Answer from the drawing. Dimensions are ordinates in mm from the lowest x, y and z of the part. Round coordinates to 2 decimals unless told otherwise and drop trailing zeros. Loops run counter-clockwise (first coordinate to the right, second up) from the corner with the lowest first, then second, coordinate; pieces in that order, holes last.
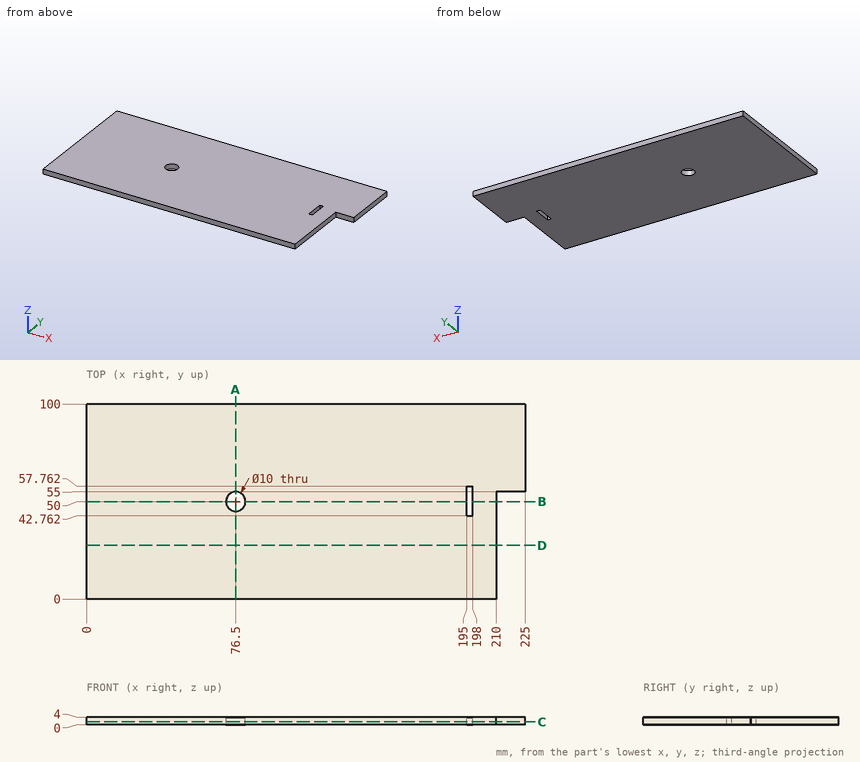
Item 1: Section D-D, the plane y = 27.5 is taken. Give the vertices of the cut face in (x, z), plus the area to 3 significant figures.
Item 2: Section C-C, the plane z = 1.6 is taken. Give the vertices of the cut face in (x, y).
Item 3: Section B-B, the plane y = 50 is taken. Give the vertices of the cut face in (x, z), plus the area to 3 significant figures.
Item 4: Section A-A, the plane x = 76.5 is taken. Give the vertices of the cut face in (y, z), plus the area to 3 significant figures.
Item 5: Each of these flat-tipped pins is pushed along its axis until it touches: P1, Ø1.2, axis at x = 214, z = 1.5, coming from the -Y side; P2, Ø2, axis at y = 14.5, z = 2.5, coming from the +X side. Where does it stop, or does it pass through?
Item 6: Straight lines are drawn through the part: line 1 (Y direction, x = 76.5, z = 2.8); line 2 (X direction, y = 19, z = 2.1); line 3 (X direction, y = 56, z = 3.8). For each, find the intervals that lie inside material, in ascending order.
Answer below:
1. outline: (0, 0) - (210, 0) - (210, 4) - (0, 4) - close
1. area: 840 mm2
2. outline: (0, 0) - (210, 0) - (210, 55) - (225, 55) - (225, 100) - (0, 100) - close; hole circle Ø10 at (76.5, 50); hole (195, 42.76) - (198, 42.76) - (198, 57.76) - (195, 57.76) - close
3. outline: (0, 0) - (71.5, 0) - (71.5, 4) - (0, 4) - close; (81.5, 0) - (195, 0) - (195, 4) - (81.5, 4) - close; (198, 0) - (210, 0) - (210, 4) - (198, 4) - close
3. area: 788 mm2
4. outline: (0, 0) - (45, 0) - (45, 4) - (0, 4) - close; (55, 0) - (100, 0) - (100, 4) - (55, 4) - close
4. area: 360 mm2
5. P1: stops at y = 55
5. P2: stops at x = 210
6. line 1: y = 0 to 45, 55 to 100
6. line 2: x = 0 to 210
6. line 3: x = 0 to 195, 198 to 225
